Check sheet for the drawn part. Datum: minimum x, y, z corner. Units: mm. Give positions to 0.01 mm unless a question says otherwise; leave off trailing zeros. Write each loop counter-clockwise with the first axis right and the second up, starting at its lowest first coordinate (ties: lowest second). Pieces come first, ordered by that corner, then holes. Notation, with made-up numbers: (33.25, -35.75) - (49.25, -35.75) arc R10 cw to (49.25, -16.75) - close; hole circle Ø11 at (-40, 29.5). An arc over 180 degrees is marked (long way). Answer as a JSON object with one key per item and string values. Group by question number.
Item 1: Scan lines: line 1 along Z through (x, y) = (7.25, 231) (1 decimal); line 2 along X through (y, z) = (109, 6) (1 decimal); line 3 along Z through (x, y) = (16, 232.5). Record each from-to range of solid material in increasing order. Write a range as [from, to].
Item 2: Draft check along Z on the marked faces 1 and 2. Enter one of: +Z half, -Z half, draft (parallel to the pull), parting line (faces both ways), or undercut.
Item 3: Sectioned sample at A-A, the plane x = 5. Record the boundary of the cut face in (y, z) (1 decimal), and give its area (3 significant figures).
Item 4: Sectioned sample at B-B, the plane y = 18.5. Record the boundary of the cut face in (x, z) (1 decimal), and give its area (3 significant figures).
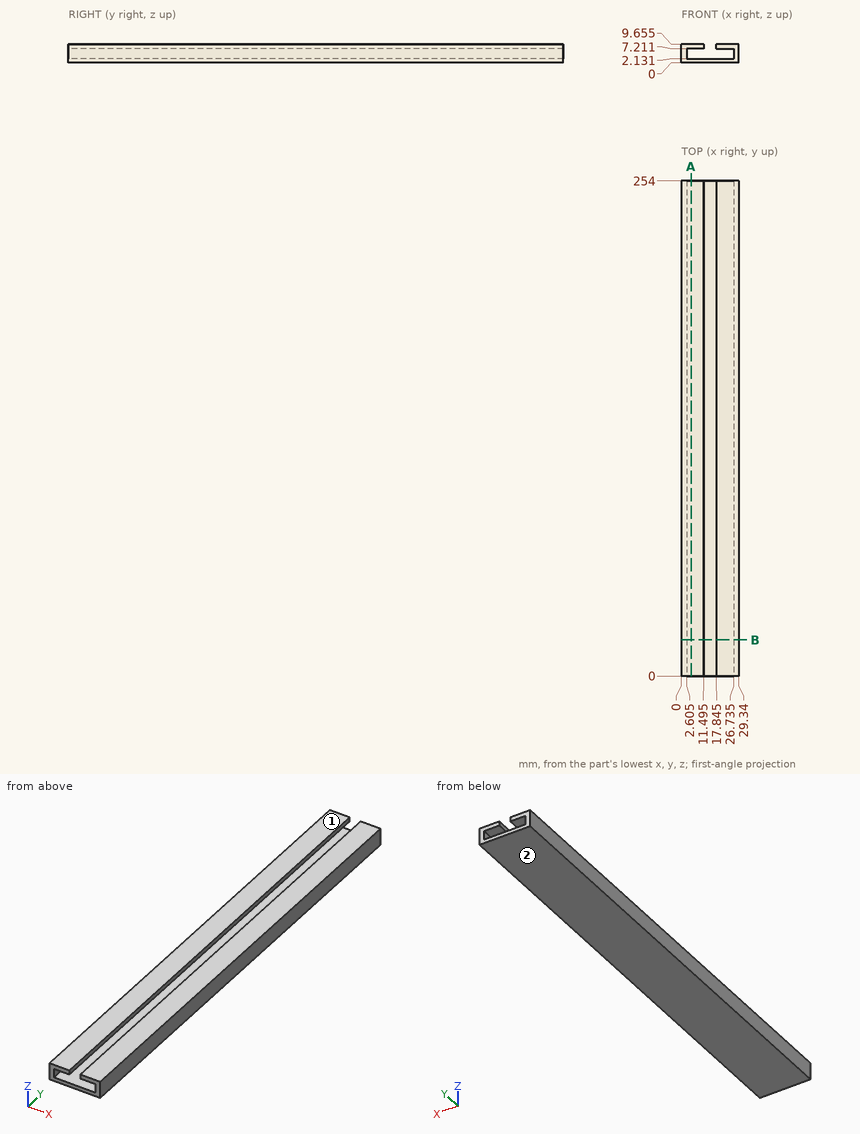
Geometry check:
{
 "1": {"line 1": "[0, 2.1], [7.2, 9.7]", "line 2": "[0, 2.6], [26.7, 29.3]", "line 3": "[0, 2.13]"},
 "2": {"face 1": "+Z half", "face 2": "-Z half"},
 "3": {"outline": "(0, 0) - (254, 0) - (254, 2.1) - (0, 2.1) - close; (0, 7.2) - (254, 7.2) - (254, 9.7) - (0, 9.7) - close", "area": "1,160 mm^2"},
 "4": {"outline": "(0, 0) - (29.3, 0) - (29.3, 9.7) - (17.8, 9.7) - (17.8, 7.2) - (26.7, 7.2) - (26.7, 2.1) - (2.6, 2.1) - (2.6, 7.2) - (11.5, 7.2) - (11.5, 9.7) - (0, 9.7) - close", "area": "145 mm^2"}
}
